Check sheet for the modelled part. Datum: model origin and axes. Units: mm. Face numbers are marked on the shaded views. Round coordinates to 2 decimals unless told otherwise and drop trailing zeros. Write each loop counter-clockwise with the first axis right and the second up, starting at its lowest first coordinate (ties: lowest second). Pieces come first, ordered by that corner, then holes. Notation, with made-up numbers: (56.5, 69.25) -> (66.5, 69.25) arc R15 cw to (66.5, 76.25) -> close; hole circle Ø8 at (14, 89.25). An arc over 180 degrees is marked (long way). One line per item, written item: value.
from build123d import *

# Parameters (mm, degrees)
SKETCH1_R               = 100
SKETCH1_R_2             = 99.238
BOSS_EXTRUDE1_DEPTH     = 27.7
F_2_5MM_DOWEL_HOLE1_D   = 2.5
F_2_5MM_DOWEL_HOLE2_D   = 2.5
SKETCH6_W               = 7.35
SKETCH6_H               = 16
CUT_EXTRUDE1_DEPTH      = 145.108605038
CUT_EXTRUDE2_DEPTH      = 145.108605038
CUT_EXTRUDE2_DEPTH_BACK = 145.108605038
SKETCH7_W               = 7.35
SKETCH7_H               = 16


with BuildPart() as part:
    # Sketch1 → Boss-Extrude1 (new body)
    with BuildSketch(Plane(origin=(0, 0, 0), x_dir=(0, 0, -1), z_dir=(1, 0, 0))):
        Circle(SKETCH1_R)
        Circle(SKETCH1_R_2, mode=Mode.SUBTRACT)
    extrude(amount=BOSS_EXTRUDE1_DEPTH)

    # Ø2.5mm Dowel Hole1 (through all)
    with Locations(Plane.XY.offset(100)):
        with Locations((24.525, 0), (3.175, 0)):
            Hole(F_2_5MM_DOWEL_HOLE1_D / 2)

    # Ø2.5mm Dowel Hole2 (through all)
    with Locations(Plane(origin=(0, 100, 0), x_dir=(1, 0, 0), z_dir=(0, 1, 0))):
        with Locations((24.525, 0), (3.175, 0)):
            Hole(F_2_5MM_DOWEL_HOLE2_D / 2)

    # Sketch6 → Cut-Extrude1 (cut, through all)
    with BuildSketch(Plane(origin=(0, 0, 0), x_dir=(-1, 0, 0), z_dir=(0, 0.7071067811865475, -0.7071067811865477))):
        with Locations((-24.525, 0)):
            Rectangle(SKETCH6_W, SKETCH6_H)
    extrude(amount=-CUT_EXTRUDE1_DEPTH, mode=Mode.SUBTRACT)

    # Sketch7 → Cut-Extrude2 (cut, two sides: drawn at the far end of the back side and taken through both)
    with BuildSketch(Plane(origin=(0, 0, 0), x_dir=(-1, 0, 0), z_dir=(0, 0.7071067811865476, 0.7071067811865476)).offset(-CUT_EXTRUDE2_DEPTH_BACK)):
        with Locations((-24.525, 0)):
            Rectangle(SKETCH7_W, SKETCH7_H)
    extrude(amount=CUT_EXTRUDE2_DEPTH + CUT_EXTRUDE2_DEPTH_BACK, mode=Mode.SUBTRACT)


solid = part.part
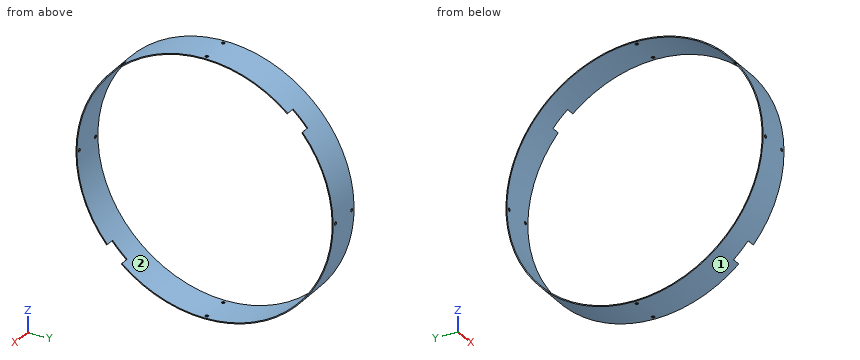
Item 1: Thickness scan on line 1 (X direction, y = 0, z = -99.55) (3 decimals); line 2 (Z direction, x = 13.5, y = 1.5); line 3 (Y direction, x = 1.75, z = -2). Record the ranges inside material, lowest first.
Answer:
line 1: x = 0 to 1.925, 4.425 to 23.275, 25.775 to 27.7
line 2: z = -99.99 to -99.23, 99.23 to 99.99
line 3: y = -99.98 to -99.22, 99.22 to 99.98
Item 2: Sectioned sample at A-A on z = 46. Enter the section's corners in (x, y), and give its area (3 significant figures).
Answer:
outline: (0, -88.79) -> (27.7, -88.79) -> (27.7, -87.93) -> (0, -87.93) -> close; (0, 87.93) -> (27.7, 87.93) -> (27.7, 88.79) -> (0, 88.79) -> close
area: 47.6 mm^2
Item 3: Sectioned sample at B-B on y = -45. Enter the section's corners in (x, z).
Answer:
outline: (0, -89.3) -> (27.7, -89.3) -> (27.7, -88.45) -> (0, -88.45) -> close; (0, 88.45) -> (27.7, 88.45) -> (27.7, 89.3) -> (0, 89.3) -> close
Item 4: Mould release check, pull along Y, two halves, no side actions. Record for the marked faces 1 and 2: pulls with the +Y half, pulls with the -Y half, needs draft (parallel to the pull), parting line crosses it, or undercut.
Answer:
face 1: parting line crosses it
face 2: undercut
Item 5: Depth check by flat-ended pin: P1, Ø6, axis at x = 8, y = 58, coming from the -Z side; P2, Ø13, axis at y = -72.5, z = 73, coming from the +X side; P3, Ø4, axis at x = 12, z = -32.5, coming from the -Y side. Enter the tip coordinate at first touch or a pass-through.
Answer:
P1: stops at z = -83.52
P2: stops at x = 20.85
P3: stops at y = -95.24
